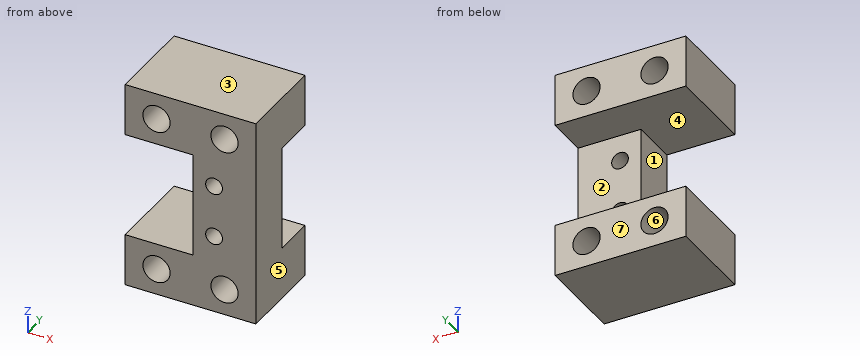
Autodesk Inventor part; units mm, degrees
ref_plane "YZ Plane" through (0, 0, 0) normal (1, 0, 0) x (0, 1, 0)
ref_plane "XZ Plane" through (0, 0, 0) normal (0, 1, 0) x (-1, 0, 0)
ref_plane "XY Plane" through (0, 0, 0) normal (0, 0, 1) x (1, 0, 0)
sketch "Sketch1" plane through (0, 0, 0) normal (0, 1, 0) x (-1, 0, 0)
  line L0 (0, 0) -> (0, -10)
  line L1 (0, 0) -> (0, 10)
  line L2 (0, 10) -> (13, 10)
  line L3 (13, 10) -> (13, 20)
  line L4 (13, 20) -> (-12, 20)
  line L5 (0, -10) -> (13, -10)
  line L6 (13, -10) -> (13, -20)
  line L7 (13, -20) -> (-12, -20)
  line L8 (-12, -20) -> (-12, 20)
  line L9 (-12, 15) -> (-6, 15)
  line L10 (13, 15) -> (7, 15)
  line L11 (13, -15) -> (7, -15)
  line L12 (-12, -15) -> (-6, -15)
  circle A0 centre (7, 15) radius 2.6
  circle A1 centre (-6, 15) radius 2.6
  circle A2 centre (-6, -15) radius 2.6
  circle A3 centre (7, -15) radius 2.6
  line L13 (0, 0) -> (-4, 0)
  line L14 (-4, 0) -> (-4, -5)
  line L15 (-4, 0) -> (-4, 5)
  circle A4 centre (-4, 5) radius 1.6
  circle A5 centre (-4, -5) radius 1.6
  line L16 (0, 10) -> (-12, 10)
  line L17 (0, -10) -> (-12, -10)
  line L18 (13, -15) -> (9.6, -15)
  line L19 (-8.6, -15) -> (-12, -15)
  line L20 (13, 15) -> (9.6, 15)
  line L21 (-8.6, 15) -> (-12, 15)
  dimension "d12" = 5.2
  dimension "d13" = 5.2
  dimension "d14" = 5.2
  dimension "d15" = 5.2
  dimension "d0" = 10
  dimension "d1" = 10
  dimension "d2" = 13
  dimension "d3" = 10
  dimension "d4" = 25
  dimension "d5" = 13
  dimension "d6" = 10
  dimension "d7" = 25
  dimension "d8" = 6
  dimension "d9" = 6
  dimension "d10" = 6
  dimension "d11" = 6
  dimension "d16" = 4
  dimension "d17" = 5
  dimension "d18" = 5
  dimension "d19" = 3.2
  dimension "d20" = 3.2
extrude "Extrusion1" add sketch "Sketch1" along normal blind 17 contours L5 L6 L7 L8 L17 | L16 L8 L4 L3 L2
extrude "Extrusion2" add sketch "Sketch1" along normal blind 9 contours L0 L17 L8 L16 L1
properties part number "servo_clip_holder1_final"
The listing builds one solid part. Answer for the finished solid, in the listing's coordinates (mm). Face numbers are marked on the shaded views. A direction names the side the tool comes from. Give positions to 0.01 mm unless a question says otherwise; leave off trailing zeros. Order: outer loops, then holes, each group sorted by start corner. A loop starts at its lowest first (then second) coordinate and runs counter-clockwise, first axis right, second up. Notation, with made-up numbers: M -19.5,2.25 L 16.5,2.25 A19 cw 16.5,22.25 Z; hole C -37,36 d1. An arc over 180 degrees is marked long. Put each result on its own line as item: value. Start each with the question number.
Item 1: Which of the six approach directions +Z, -Z, +X, -X, +Y, -Y give full straight-line access (tool end or side, diameter ignored) to the marked faces 1, 2, 3 and 4?
Item 2: The part is cut by section D-D, the plane z = -5. Determine the outline of the cut face in (x, y).
Item 3: For a pull along X with two mould halves and no side action, classify the marked faces 5, 6 and 7 as +X half, -X half, draft (parallel to the pull), parting line (faces both ways), or undercut.
Item 4: Find the intervals of material crossed by line 1 along Z through (x, y) = (6, 10.5); line 2 along Z through (x, y) = (4, 7.25); line 3 along Z through (x, y) = (3, 1.75), in increasing order.
Item 5: The part is cut by section B-B, the plane y = 11.25. Determine the outline of the cut face in (x, z), and give its area (3 significant figures).
Item 6: The part is cut by section A-A, the plane z = 15. Determine the outline of the cut face in (x, y).
Item 7: Flat-ended cylindrical pins translate along their axes: P1, Ø7, axis at x = 6, z = -15, coming from the -Y side; P2, Ø3.5, axis at x = 4, z = 5, coming from the +Y side; P3, Ø7, axis at y = 6, z = -2, coming from the -X side. Find the tip coordinate at first contact, or state that the pin passes through.
Item 8: The part is cut by section C-C, the plane x = -10.25. Determine the outline of the cut face in (y, z), and give its area (3 significant figures).
Answer key:
1. face 1: -X, +Y, -Y
1. face 2: +X, -X, +Y
1. face 3: +Z, +X, -X, +Y, -Y
1. face 4: -X, +Y
2. outline: M 0,0 L 2.4,0 L 2.4,9 L 0,9 Z; M 5.6,0 L 12,0 L 12,9 L 5.6,9 Z
3. face 5: +X half
3. face 6: undercut
3. face 7: draft
4. line 1: z = -20 to -17.6, -12.4 to -10, 10 to 12.4, 17.6 to 20
4. line 2: z = -20 to -16.66, -13.34 to -6.6, -3.4 to 3.4, 6.6 to 13.34, 16.66 to 20
4. line 3: z = -20 to -6.25, -3.75 to 3.75, 6.25 to 20
5. outline: M -13,-20 L 12,-20 L 12,-10 L -13,-10 Z; M -13,10 L 12,10 L 12,20 L -13,20 Z; hole C -7,-15 d5.2; hole C -7,15 d5.2; hole C 6,-15 d5.2; hole C 6,15 d5.2
5. area: 415 mm²
6. outline: M -13,0 L -9.6,0 L -9.6,17 L -13,17 Z; M -4.4,0 L 3.4,0 L 3.4,17 L -4.4,17 Z; M 8.6,0 L 12,0 L 12,17 L 8.6,17 Z
7. P1: stops at y = 0
7. P2: stops at y = 9
7. P3: stops at x = 0
8. outline: M 0,-20 L 17,-20 L 17,-10 L 0,-10 Z; M 0,10 L 17,10 L 17,20 L 0,20 Z
8. area: 340 mm²
